Geometry: see drawing. Coordinates: mm, zero at the bounding-box minimum. Give positions to 0.01 mm unless a question says otherwise; leave off trailing zeros. Loops run counter-clockwise (first coordinate to the right, second up) from the corner with the lowest first, then second, coordinate; pieces in that order, holes last. Notation, with made-up numbers: (10.5, -6) - (53.5, -6) arc R11 cw to (53.5, 15) - close; hole circle Ø5 at (-4, 56). An arc over 180 degrees is marked (long way). Use one line per item in the form item = value.
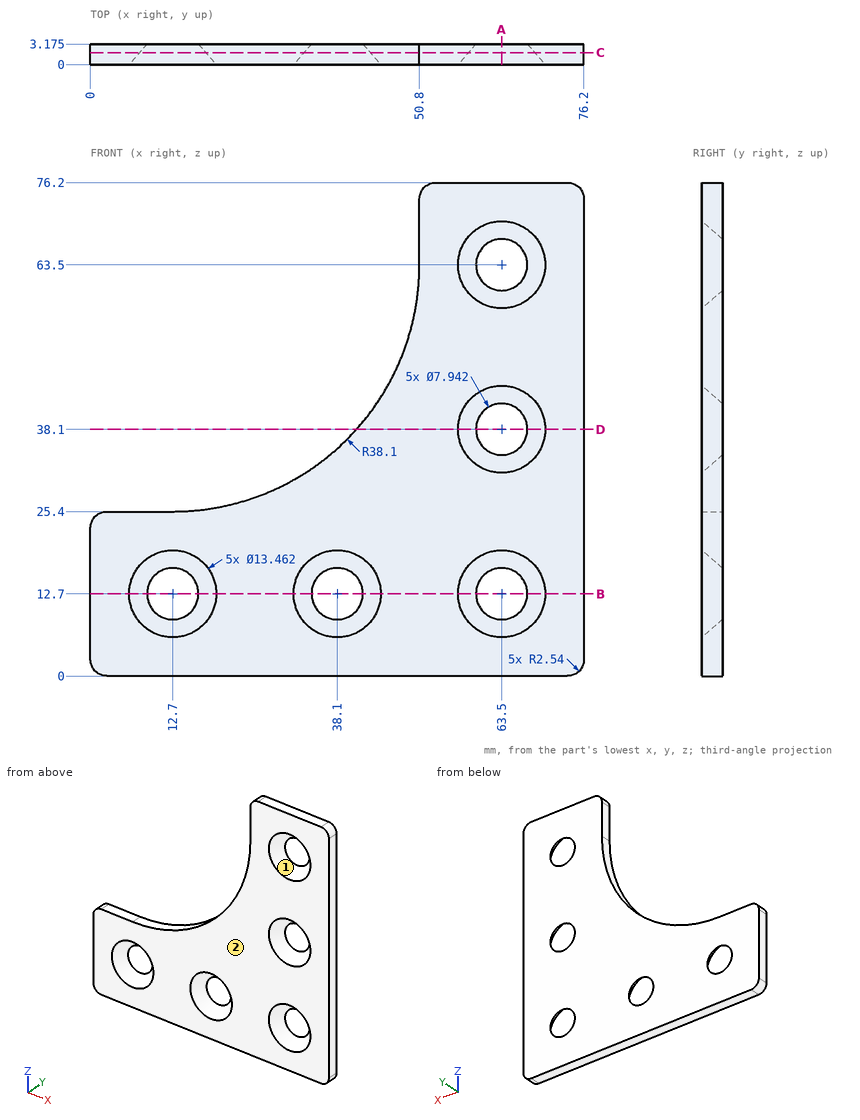
(1) Cut plane B-B (z = 12.7). Return the cut outline in (x, y) (3 decimals).
Solution:
outline = (0, 0) - (5.969, 0) - (8.729, 3.175) - (0, 3.175) - close; (16.671, 3.175) - (19.431, 0) - (31.369, 0) - (34.129, 3.175) - close; (42.071, 3.175) - (44.831, 0) - (56.769, 0) - (59.529, 3.175) - close; (67.471, 3.175) - (70.231, 0) - (76.2, 0) - (76.2, 3.175) - close
(2) Cut plane D-D (z = 38.1). Return the cut outline in (x, y) (3 decimals).
Solution:
outline = (41.098, 0) - (56.769, 0) - (59.529, 3.175) - (41.098, 3.175) - close; (67.471, 3.175) - (70.231, 0) - (76.2, 0) - (76.2, 3.175) - close
(3) Material intervals for L1, parallel to X at y = 1.55, z = 17; L2, parallel to X at y = 1.8, z = 37.5; L3, parallel to Z at x = 40, y = 1, sorted ascending. Write a range as from..to.
Solution:
L1 = 0..9.46, 15.94..34.86, 41.34..60.26, 66.74..76.2
L2 = 40.55..58.37, 68.63..76.2
L3 = 0..7.15, 18.25..36.92
(4) Pin query (flat end, axial travel): P1, Ø1, axis at x = 7.5, y = 1.5, coming from the +Z side; P2, Ø1, axis at y = 1, z = 71, coming from the -X side. Return the tip coordinate at first contact, or that it passes through.
Solution:
P1 = 25.4
P2 = 50.8
(5) Cut plane C-C (y = 1.85). Return the cut outline in (x, z), plus the area to 3 significant figures.
Solution:
outline = (0, 2.54) arc R2.54 ccw to (2.54, 0) - (73.66, 0) arc R2.54 ccw to (76.2, 2.54) - (76.2, 73.66) arc R2.54 ccw to (73.66, 76.2) - (53.34, 76.2) arc R2.54 ccw to (50.8, 73.66) - (50.8, 63.5) arc R38.1 cw to (12.7, 25.4) - (2.54, 25.4) arc R2.54 ccw to (0, 22.86) - close; hole circle Ø10.25 at (12.7, 12.7); hole circle Ø10.25 at (38.1, 12.7); hole circle Ø10.25 at (63.5, 12.7); hole circle Ø10.25 at (63.5, 38.1); hole circle Ø10.25 at (63.5, 63.5)
area = 3,120 mm2
(6) Pull-direction query (X, two-part tool) for the marked faces 1 and 2; classes: released by +X, released by -X, zero draft, split by the parting line, or undercut.
Solution:
face_1 = undercut
face_2 = zero draft
(7) Cut plane A-A (x = 63.5). Return the cut outline in (y, z) (3 decimals), plus the area to 3 significant figures.
Solution:
outline = (0, 0) - (3.175, 0) - (3.175, 8.729) - (0, 5.969) - close; (0, 19.431) - (3.175, 16.671) - (3.175, 34.129) - (0, 31.369) - close; (0, 44.831) - (3.175, 42.071) - (3.175, 59.529) - (0, 56.769) - close; (0, 70.231) - (3.175, 67.471) - (3.175, 76.2) - (0, 76.2) - close
area = 140 mm2
